Check sheet for the drawn part. Datum: minimum x, y, z corner. Units: mm. A direction names the side the tool comes from. Give positions to 0.01 mm unless a question says otherwise; leave off trailing zeros. Order: outer loops, then holes, each group sorted by start corner. A loop starts at its lowest first (then second) coordinate and runs counter-clockwise, first axis right, second up. Notation, with made-up numbers: (18, 31) -> (46, 31) arc R24 cw to (46, 45) -> close; hole circle Ø5 at (51.5, 47). An arc over 180 degrees is marked (long way). One line per question, with ' | ' between items. Start each with the question number.
Q1. Section check D-D on y = 27.5. Record the cut outline in (x, z), plus the area to 3 significant figures.
Q2. Section check A-A on z = 15.5. Record the cut outline in (x, y).
Q3. Access from +Z, -Z, +X, -X, +Y, -Y to the whole of each face (thin tool, end or side, straight path). Record for the marked faces 5, 6 and 7.
Q4. Go/stop test with flat-tipped pins: pin 1 (1 mm diameter, centred on y = 18.5, z = 12, fed in from -X); pin 2 (4.5 mm diameter, centred on y = 23, z = 9.5, fed in from +X); pin 3 (10 mm diameter, centred on x = 43, z = 16.5, fed in from -Y); pin 4 (6 mm diameter, centred on x = 7.5, y = 7.5, fed in from +Z). Record where each tip stops, or that it passes through.
Q5. Material ranges on probe 1 along X at (y, z) = (32, 8); probe 2 along Y at (x, z) = (47.5, 2.05); probe 3 along Y at (x, z) = (27.5, 3.6), recorded low to high. Write a range as [from, to].
Q6. Mould release check, pull along X, two halves, no side actions. Record for the marked faces 1, 2, 3 and 4: released by +X, released by -X, zero draft, split by the parting line, or undercut.
Q7. Section check B-B on y = 7.5. Record the cut outline in (x, z), plus the area to 3 significant figures.
Q8. Section check C-C on x = 27.5. Record the cut outline in (y, z).
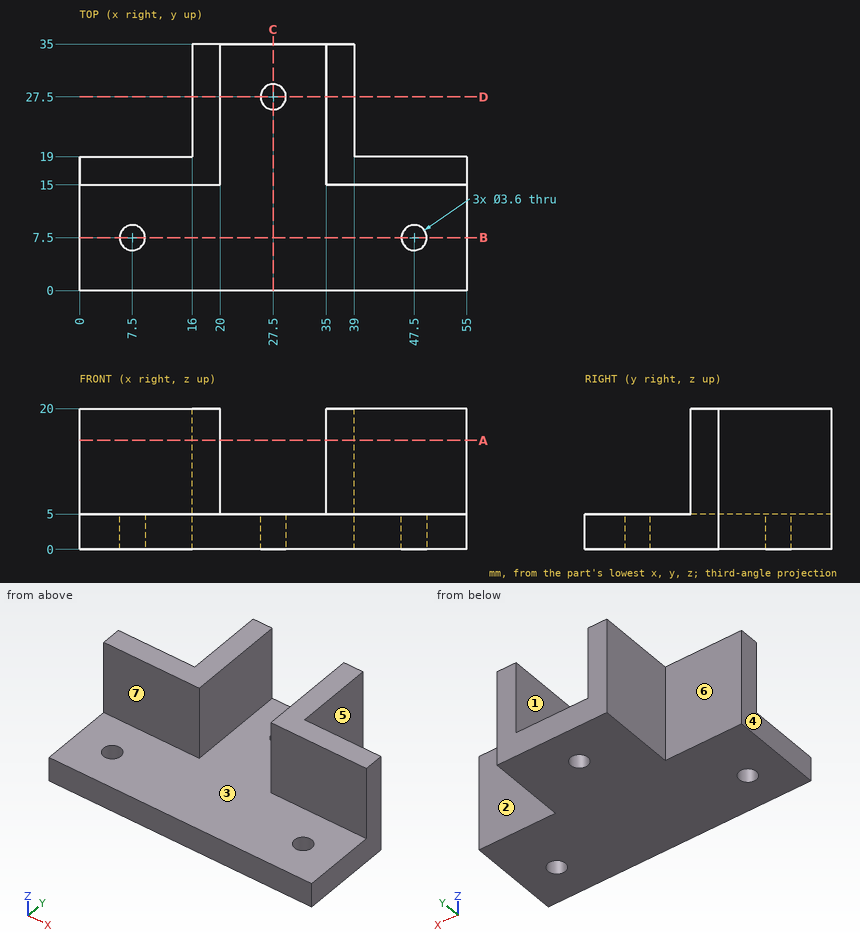
Filled in:
1) outline: (16, 0) -> (25.7, 0) -> (25.7, 5) -> (20, 5) -> (20, 20) -> (16, 20) -> close; (29.3, 0) -> (39, 0) -> (39, 20) -> (35, 20) -> (35, 5) -> (29.3, 5) -> close | area: 217 mm²
2) outline: (0, 15) -> (20, 15) -> (20, 35) -> (16, 35) -> (16, 19) -> (0, 19) -> close; (35, 15) -> (55, 15) -> (55, 19) -> (39, 19) -> (39, 35) -> (35, 35) -> close
3) face 5: +Z, -Z, +X, +Y | face 6: +Z, -Z, -X, +Y | face 7: +Z, +X, -X, -Y
4) pin 1: x = 0 | pin 2: x = 39 | pin 3: y = 15 | pin 4: z = 5
5) probe 1: [16, 20], [35, 39] | probe 2: [0, 5.7], [9.3, 19] | probe 3: [0, 25.7], [29.3, 35]
6) face 1: undercut | face 2: zero draft | face 3: undercut | face 4: released by -X
7) outline: (0, 0) -> (5.7, 0) -> (5.7, 5) -> (0, 5) -> close; (9.3, 0) -> (45.7, 0) -> (45.7, 5) -> (9.3, 5) -> close; (49.3, 0) -> (55, 0) -> (55, 5) -> (49.3, 5) -> close | area: 239 mm²
8) outline: (0, 0) -> (25.7, 0) -> (25.7, 5) -> (0, 5) -> close; (29.3, 0) -> (35, 0) -> (35, 5) -> (29.3, 5) -> close
